Geometry check sheet. Reference: the model listing, model coordinates, mm. Face numbers are marked on the shaded views. A direction names the side the tool comes from. Round coordinates to 2 decimals unless told otherwise and drop trailing zeros. Order: outer loops, then holes, each group sorted by start corner. A loop starts at its lowest first (then second) coordinate and runs counter-clockwise, first axis right, second up. Notation, with made-up numbers: (72, 13) - (131, 13) arc R20 ccw to (131, 31) - close; hole circle Ø5 at (-23.75, 8.5). An arc over 180 degrees is marked (long way). Answer as CSV lines item,"result". Start each with the question number.
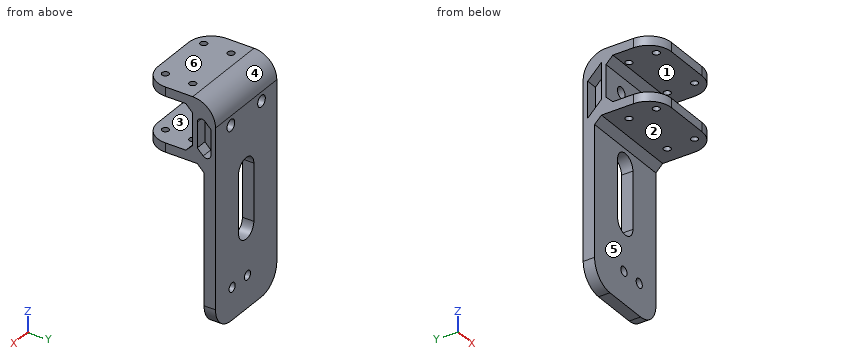
```python
from build123d import *

# Parameters (mm, degrees)
SKETCH_1_W          = 40
SKETCH_1_H          = 28
EXTRUDE_1_DEPTH     = 10
SKETCH_2_W          = 40
SKETCH_2_H          = 4
EXTRUDE_2_DEPTH     = 10
SKETCH_4_W          = 40
SKETCH_4_H          = 5
EXTRUDE_3_DEPTH     = 15
SKETCH_6_W          = 40
SKETCH_6_H          = 5
EXTRUDE_4_DEPTH     = 15
SKETCH_8_R          = 2.5
CUT_EXTRUDE_2_DEPTH = 15
CHAMFER_1_SIZE      = 3
FILLET_1_R          = 10
CHAMFER_2_SIZE      = 3
SKETCH_9_R          = 1.5
CUT_EXTRUDE_3_DEPTH = 38.416573868
CUT_EXTRUDE_4_DEPTH = 5
FILLET_3_R          = 2
SKETCH_11_W         = 40
SKETCH_11_H         = 7
EXTRUDE_5_DEPTH     = 3
CHAMFER_3_SIZE      = 1
SKETCH_12_W         = 40
SKETCH_12_H         = 5
EXTRUDE_6_DEPTH     = 30
SKETCH_13_R         = 2
CUT_EXTRUDE_5_DEPTH = 30
SKETCH_16_W         = 20
SKETCH_16_H         = 6.386072782
CUT_EXTRUDE_6_DEPTH = 85.711274338
SKETCH_17_W         = 40
SKETCH_17_H         = 4
EXTRUDE_8_DEPTH     = 12
SKETCH_18_R         = 1.5
CUT_EXTRUDE_7_DEPTH = 93.887028158
CUT_EXTRUDE_8_DEPTH = 84.066238629
SKETCH_21_W         = 40
SKETCH_21_H         = 5
EXTRUDE_9_DEPTH     = 10
FILLET_5_R          = 10


with BuildPart() as part:
    # 草图1 → 凸台-拉伸1 (new body)
    with BuildSketch(Plane(origin=(0, 0, 0), x_dir=(1, 0, 0), z_dir=(0, 1, 0))):
        Rectangle(SKETCH_1_W, SKETCH_1_H)
    extrude(amount=EXTRUDE_1_DEPTH)

    # 草图2 → 凸台-拉伸2 (add)
    with BuildSketch(Plane.XZ):
        with Locations((0, 12)):
            Rectangle(SKETCH_2_W, SKETCH_2_H)
        with Locations((0, -12)):
            Rectangle(SKETCH_2_W, SKETCH_2_H)
    extrude(amount=EXTRUDE_2_DEPTH)

    # 草图4 → 凸台-拉伸3 (add)
    with BuildSketch(Plane(origin=(0, 0, -14), x_dir=(-1, 0, 0), z_dir=(0, 0, -1))):
        with Locations((0, 7.5)):
            Rectangle(SKETCH_4_W, SKETCH_4_H)
    extrude(amount=EXTRUDE_3_DEPTH)

    # 草图6 → 凸台-拉伸4 (add)
    with BuildSketch(Plane(origin=(0, 0, -29), x_dir=(-1, 0, 0), z_dir=(0, 0, -1))):
        with Locations((0, 7.5)):
            Rectangle(SKETCH_6_W, SKETCH_6_H)
    extrude(amount=EXTRUDE_4_DEPTH)

    # 草图8 → 切除-拉伸2 (cut)
    with BuildSketch(Plane(origin=(0, 10, 0), x_dir=(1, 0, 0), z_dir=(0, 1, 0))):
        with Locations(Location((-10, 0, 0), (0, 0, 270))):
            Circle(SKETCH_8_R)
        with Locations(Location((10, 0, 0), (0, 0, 270))):
            Circle(SKETCH_8_R)
    extrude(amount=-CUT_EXTRUDE_2_DEPTH, mode=Mode.SUBTRACT)

    # 倒角1
    chamfer_1_edges = [part.edges().sort_by_distance(p)[0] for p in [
        (0, 0, 10),
        (0, 0, -10),
    ]]
    chamfer(chamfer_1_edges, length=CHAMFER_1_SIZE)

    # 圆角1
    fillet_1_edges = [part.edges().sort_by_distance(p)[0] for p in [
        (0, 10, 14),
    ]]
    fillet(fillet_1_edges, radius=FILLET_1_R)

    # 倒角2
    chamfer_2_edges = [part.edges().sort_by_distance(p)[0] for p in [
        (0, 5, -14),
    ]]
    chamfer(chamfer_2_edges, length=CHAMFER_2_SIZE)

    # 草图9 → 切除-拉伸3 (cut, through all)
    with BuildSketch(Plane(origin=(0, 0, -14), x_dir=(-1, 0, 0), z_dir=(0, 0, -1))):
        with Locations((-12.5, -5)):
            Circle(SKETCH_9_R)
        with Locations((12.5, -5)):
            Circle(SKETCH_9_R)
    extrude(amount=-CUT_EXTRUDE_3_DEPTH, mode=Mode.SUBTRACT)

    # 草图10 → 切除-拉伸4 (cut)
    with BuildSketch(Plane(origin=(20, 0, 0), x_dir=(0, 0, -1), z_dir=(1, 0, 0))):
        Polygon((-2.618541417, 8), (-8.618541417, 2), (7.264071942, 2), (13.264071942, 8), align=None)
    cut_extrude_4 = extrude(amount=-CUT_EXTRUDE_4_DEPTH, mode=Mode.SUBTRACT)

    # 圆角3
    fillet_3_edges = [part.edges().sort_by_distance(p)[0] for p in [
        (17.5, 8, -13.264071942),
        (17.5, 2, 8.618541417),
    ]]
    fillet(fillet_3_edges, radius=FILLET_3_R)

    # 镜向1: 切除-拉伸4 across plane
    add(cut_extrude_4.mirror(Plane(origin=(0, 0, 0), x_dir=(0, 0, 1), z_dir=(1, 0, 0))), mode=Mode.SUBTRACT)

    # 草图11 → 凸台-拉伸5 (add)
    with BuildSketch(Plane.XZ.offset(10)):
        with Locations((0, -10.5)):
            Rectangle(SKETCH_11_W, SKETCH_11_H)
        with Locations((0, 10.5)):
            Rectangle(SKETCH_11_W, SKETCH_11_H)
    extrude(amount=-EXTRUDE_5_DEPTH)

    # 倒角3
    chamfer_3_edges = [part.edges().sort_by_distance(p)[0] for p in [
        (0, -7, -7),
        (0, -7, 7),
    ]]
    chamfer(chamfer_3_edges, length=CHAMFER_3_SIZE)

    # 草图12 → 凸台-拉伸6 (add)
    with BuildSketch(Plane(origin=(0, 0, -44), x_dir=(-1, 0, 0), z_dir=(0, 0, -1))):
        with Locations((0, 7.5)):
            Rectangle(SKETCH_12_W, SKETCH_12_H)
    extrude(amount=EXTRUDE_6_DEPTH)

    # 草图13 → 切除-拉伸5 (cut)
    with BuildSketch(Plane(origin=(0, 10, 0), x_dir=(1, 0, 0), z_dir=(0, 1, 0))):
        with Locations(Location((9.14, 70, 0), (0, 0, 270))):
            Circle(SKETCH_13_R)
        with Locations(Location((-0.86, 70, 0), (0, 0, 270))):
            Circle(SKETCH_13_R)
    extrude(amount=-CUT_EXTRUDE_5_DEPTH, mode=Mode.SUBTRACT)

    # 草图16 → 切除-拉伸6 (cut, through all)
    with BuildSketch(Plane(origin=(20, 0, 0), x_dir=(0, 0, -1), z_dir=(1, 0, 0))):
        with Locations((0, -10.193036391)):
            Rectangle(SKETCH_16_W, SKETCH_16_H)
    extrude(amount=-CUT_EXTRUDE_6_DEPTH, mode=Mode.SUBTRACT)

    # 草图17 → 凸台-拉伸8 (add)
    with BuildSketch(Plane.XZ.offset(10)):
        with Locations((0, -12)):
            Rectangle(SKETCH_17_W, SKETCH_17_H)
        with Locations((0, 12)):
            Rectangle(SKETCH_17_W, SKETCH_17_H)
    extrude(amount=EXTRUDE_8_DEPTH)

    # 草图18 → 切除-拉伸7 (cut, through all)
    with BuildSketch(Plane.XY.offset(14)):
        with Locations(Location((12.5, -5, 0), (0, 0, 180))):
            Circle(SKETCH_18_R)
        with Locations(Location((-12.5, -5, 0), (0, 0, 180))):
            Circle(SKETCH_18_R)
        with Locations((-12.5, -17)):
            Circle(SKETCH_18_R)
        with Locations((12.5, -17)):
            Circle(SKETCH_18_R)
    extrude(amount=-CUT_EXTRUDE_7_DEPTH, mode=Mode.SUBTRACT)

    # 草图19 → 切除-拉伸8 (cut, through all)
    with BuildSketch(Plane(origin=(0, 10, 0), x_dir=(1, 0, 0), z_dir=(0, 1, 0))):
        with BuildLine():
            Line((5, 49), (5, 24))
            ThreePointArc((5, 24), (0, 19), (-5, 24))
            Line((-5, 24), (-5, 49))
            ThreePointArc((-5, 49), (0, 54), (5, 49))
        make_face()
    extrude(amount=-CUT_EXTRUDE_8_DEPTH, mode=Mode.SUBTRACT)

    # 草图21 → 凸台-拉伸9 (add)
    with BuildSketch(Plane(origin=(0, 0, -74), x_dir=(-1, 0, 0), z_dir=(0, 0, -1))):
        with Locations((0, 7.5)):
            Rectangle(SKETCH_21_W, SKETCH_21_H)
    extrude(amount=EXTRUDE_9_DEPTH)

    # 圆角5
    fillet_5_edges = [part.edges().sort_by_distance(p)[0] for p in [
        (-20, -22, -12),
        (20, -22, -12),
        (-20, -22, 12),
        (20, -22, 12),
        (20, 7.5, -84),
        (-20, 7.5, -84),
    ]]
    fillet(fillet_5_edges, radius=FILLET_5_R)


solid = part.part
```
1. Section check A-A on z = -36.5. Record the boundary of the cut face in (x, y), plus the area to 3 significant figures.
2. Access from +Z, -Z, +X, -X, +Y, -Y to the whole of each face (thin tool, end or side, straight path). Record for the marked faces 5 and 6.
3. Section check D-D on z = -70. Record the boundary of the cut face in (x, y), plus the area to 3 significant figures.
4. Go/stop test with flat-tipped pins: pin 1 Ø3 at (x, z) = (-10, 0) entering from +Y; pin 2 Ø3 at (x, y) = (-0.5, -6.5) entering from -Z; pin 3 Ø5.5 at (x, z) = (16.5, -4) entering from -Y; pin 4 Ø3 at (y, z) = (5, -2.5) entering from -X. Record where each tip stops, or that it passes through.
5. Section check B-B on y = -11. Record the boundary of the cut face in (x, z).
6. Draft check along Z on the marked faces 1, 2, 3 and 4. Enter one of: released by +Z, released by -Z, zero draft, split by the parting line, or undercut.
7. Section check C-C on y = -5. Record the boundary of the cut face in (x, z), plus the area to 3 significant figures.
8. Thickness scan on probe 1 along Z at (x, y) = (5, -15.5); probe 2 along X at (y, z) = (3.25, 0); probe 3 along Y at (x, z) = (-12.5, 10.85). Record the ranges inside material, lowest first.
Numbers:
1,outline,"(-20, 5) - (-5, 5) - (-5, 10) - (-20, 10) - close; (5, 5) - (20, 5) - (20, 10) - (5, 10) - close"
1,area,"150 mm2"
2,face 5,"-Z, +X, -X, -Y"
2,face 6,"+Z, +X, -X, +Y, -Y"
3,outline,"(-20, 5) - (-2.86, 5) - (-2.86, 10) - (-20, 10) - close; (1.14, 5) - (7.14, 5) - (7.14, 10) - (1.14, 10) - close; (11.14, 5) - (20, 5) - (20, 10) - (11.14, 10) - close"
3,area,"160 mm2"
4,pin 1,"passes through"
4,pin 2,"stops at z = -14"
4,pin 3,"stops at y = 0"
4,pin 4,"stops at x = -15"
5,outline,"(-20, -14) - (20, -14) - (20, -10) - (-20, -10) - close; (-20, 10) - (20, 10) - (20, 14) - (-20, 14) - close"
6,face 1,"undercut"
6,face 2,"released by -Z"
6,face 3,"undercut"
6,face 4,"released by +Z"
7,outline,"(-20, -14) - (-14, -14) - (-14, -10) - (-20, -10) - close; (-20, 10) - (-14, 10) - (-14, 14) - (-20, 14) - close; (-11, -14) - (11, -14) - (11, -10) - (-11, -10) - close; (-11, 10) - (11, 10) - (11, 14) - (-11, 14) - close; (14, -14) - (20, -14) - (20, -10) - (14, -10) - close; (14, 10) - (20, 10) - (20, 14) - (14, 14) - close"
7,area,"272 mm2"
8,probe 1,"z = -14 to -10, 10 to 14"
8,probe 2,"x = -15 to -12.5, -7.5 to 7.5, 12.5 to 15"
8,probe 3,"y = -21.68 to -18.5, -15.5 to -6.5, -3.5 to 7.29"
